For this review, use the dimensioned drawing (mm, ordinates from the lowest corner) and the shaded views. A direction names the side the tool comes from. Round coordinates to 2 decimals unless told otherwise and drop trailing zeros. Write each loop counter-clockwise with the first axis right and the second up, starting at its lowest first coordinate (ties: lowest second). Pieces come first, ordered by that corner, then holes. Notation, with made-up numbers: (72.5, 66) -> (116.5, 66) arc R21 cw to (116.5, 94) -> close; hole circle Ø2 at (48.25, -1). An arc over 180 degrees is marked (long way). Write each question's results on one line, items separated by ' | '. Start each with the question number.
Item 1: The part is to be moulded in two halves that separate along X. For the marked faces 4, 5, 6 and 7, say which applies: +X half, -X half, draft (parallel to the pull), parting line (faces both ways), or undercut.
Item 2: Add section D-D (x = 47.5). State the section outline as (y, z) points, plus the area to 3 significant figures.
Item 3: Add section C-C (x = 6.6). State the section outline as (y, z) points, plus the area to 3 significant figures.
Item 4: Add section A-A (z = 9). State the section outline as (x, y) points, plus the area to 3 significant figures.
Item 5: Tool access review of the marked faces 1, 2 and 3: name each direction out of +Z, -Z, +X, -X, +Y, -Y from which nothing blocks a thin tool from reaching the whole face with its end or side.
Item 6: Add section B-B (y = 6.6). State the section outline as (x, z) points.
Item 7: To check wall thickness, follow line 1 along Y through (x, z) = (44.6, 8.95); line 2 along Y through (x, z) = (35.5, 5.5); line 3 along X through (y, z) = (46.5, 7.25). State the ranges of each line that lie inside material, in increasing order.
Item 8: Clearance check with flat-ended pins moving along their axes: pin 1 (3.5 mm diameter, centred on x = 44, y = 45, fed in from +Z); pin 2 (8.5 mm diameter, centred on x = 22.5, y = 19.5, fed in from +Z). State where each tip first meets the part, or that it passes through.
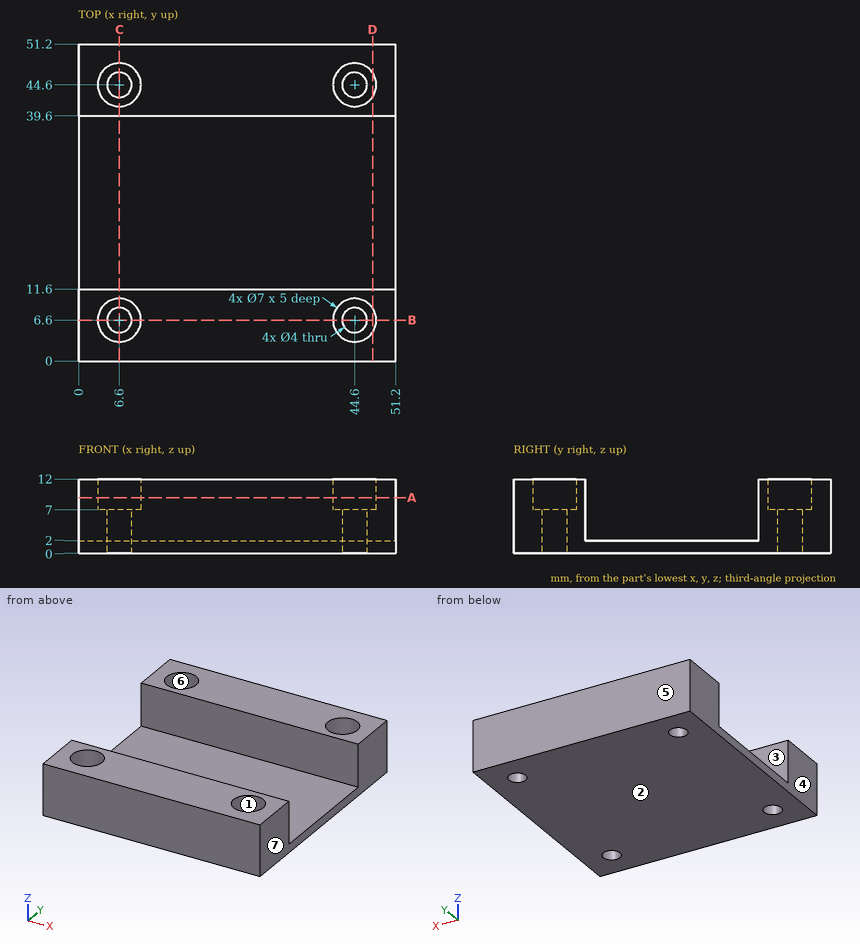
Responses:
1) face 4: -X half | face 5: draft | face 6: undercut | face 7: +X half
2) outline: (0, 0) -> (51.2, 0) -> (51.2, 12) -> (46.56, 12) -> (46.56, 7) -> (42.64, 7) -> (42.64, 12) -> (39.6, 12) -> (39.6, 2) -> (11.6, 2) -> (11.6, 12) -> (8.56, 12) -> (8.56, 7) -> (4.64, 7) -> (4.64, 12) -> (0, 12) -> close | area: 295 mm^2
3) outline: (0, 0) -> (4.6, 0) -> (4.6, 7) -> (3.1, 7) -> (3.1, 12) -> (0, 12) -> close; (8.6, 0) -> (42.6, 0) -> (42.6, 7) -> (41.1, 7) -> (41.1, 12) -> (39.6, 12) -> (39.6, 2) -> (11.6, 2) -> (11.6, 12) -> (10.1, 12) -> (10.1, 7) -> (8.6, 7) -> close; (46.6, 0) -> (51.2, 0) -> (51.2, 12) -> (48.1, 12) -> (48.1, 7) -> (46.6, 7) -> close | area: 208 mm^2
4) outline: (0, 0) -> (51.2, 0) -> (51.2, 11.6) -> (0, 11.6) -> close; (0, 39.6) -> (51.2, 39.6) -> (51.2, 51.2) -> (0, 51.2) -> close; hole circle Ø7 at (6.6, 6.6); hole circle Ø7 at (6.6, 44.6); hole circle Ø7 at (44.6, 6.6); hole circle Ø7 at (44.6, 44.6) | area: 1,030 mm^2
5) face 1: +Z | face 2: -Z, +X, -X, +Y, -Y | face 3: +Z, +X, -X
6) outline: (0, 0) -> (4.6, 0) -> (4.6, 7) -> (3.1, 7) -> (3.1, 12) -> (0, 12) -> close; (8.6, 0) -> (42.6, 0) -> (42.6, 7) -> (41.1, 7) -> (41.1, 12) -> (10.1, 12) -> (10.1, 7) -> (8.6, 7) -> close; (46.6, 0) -> (51.2, 0) -> (51.2, 12) -> (48.1, 12) -> (48.1, 7) -> (46.6, 7) -> close
7) line 1: y = 0 to 3.1, 10.1 to 11.6, 39.6 to 41.1, 48.1 to 51.2 | line 2: y = 0 to 11.6, 39.6 to 51.2 | line 3: x = 0 to 3.66, 9.54 to 41.66, 47.54 to 51.2
8) pin 1: stops at z = 7 | pin 2: stops at z = 2
